Can you work these out from the model? Positions are in its coordinate system, mm. A direction names the side the tool comes from. Round coordinates to 2 decimals unless told otherwise and drop trailing zeros. Write each loop counter-clockwise with the first axis right and the second up, starting at its lowest first coordinate (ties: lowest second). Pieces come first, ordered by that corner, then holes. Notation, with made-up numbers: M 15.25,63.25 L 30.25,63.25 A16 cw 30.25,94.25 Z; hole C 84,31.25 d3. An arc over 180 degrees is marked long. Answer as a JSON object with one key per item and string values. Group by question number.
1) Please list where these lines run through material, in increasing order: L1, parallel to Z at x = -8, y = 4.3; L2, parallel to X at y = 3.25, z = -18.5. Write a range as [from, to].
2) If we mould it in two halves opening along X, with no side actions, what happens to faces 3 (the flat face through (-113.919, 3, 1)), 4 (the flat face through (108.839, 3, 1)), 5 (the flat face through (-9, 0, 79))? For each: +X half, -X half, draft (parallel to the pull), parting line (faces both ways), or undercut.
3) Suppose I cut it at B-B, the plane z = -10. Write out the boundary of the cut face in (x, y).
4) On a 3-axis mill with a long thin cutter (end or side, diameter ignored), from which of +Z, -Z, +X, -X, +Y, -Y can I reach the whole of each face in a straight line? I mean faces 1 (the flat face through (-9, 5.08, 79)), 2 (the cylindrical face through (-107.21, 2.58, 75.55)). Say none if no direction works.
5) Suppose I cut it at A-A, the plane x = 4. Write out the boundary of the cut face in (y, z), and give its area (3 significant figures).
6) Suppose I cut it at C-C, the plane y = 4.3. Write out the boundary of the cut face in (x, z), and give its area (3 significant figures).
from build123d import *

# Parameters (mm, degrees)
SKETCH1_W      = 227.838
SKETCH1_H      = 164.338
SKETCH1_W_2    = 217.678
SKETCH1_H_2    = 154.178
EXTRUDE1_DEPTH = 5.08
FILLET1_R      = 5.4102
FILLET2_R      = 10.4902


with BuildPart() as part:
    # Sketch1 → Extrude1 (new body)
    with BuildSketch(Plane(origin=(0, 0, 0), x_dir=(1, 0, 0), z_dir=(0, 1, 0))):
        Rectangle(SKETCH1_W, SKETCH1_H)
        Rectangle(SKETCH1_W_2, SKETCH1_H_2, mode=Mode.SUBTRACT)
    extrude(amount=EXTRUDE1_DEPTH)

    # Fillet1
    fillet1_edges = [part.edges().sort_by_distance(p)[0] for p in [
        (-108.839, 2.54, -77.089),
        (-108.839, 2.54, 77.089),
        (108.839, 2.54, 77.089),
        (108.839, 2.54, -77.089),
    ]]
    fillet(fillet1_edges, radius=FILLET1_R)

    # Fillet2
    fillet2_edges = [part.edges().sort_by_distance(p)[0] for p in [
        (-113.919, 2.54, -82.169),
        (113.919, 2.54, -82.169),
        (113.919, 2.54, 82.169),
        (-113.919, 2.54, 82.169),
    ]]
    fillet(fillet2_edges, radius=FILLET2_R)


solid = part.part
Results:
{
 "1": {"L1": "[-82.17, -77.09], [77.09, 82.17]", "L2": "[-113.92, -108.84], [108.84, 113.92]"},
 "2": {"face 3": "-X half", "face 4": "undercut", "face 5": "draft"},
 "3": {"outline": "M -113.92,0 L -108.84,0 L -108.84,5.08 L -113.92,5.08 Z; M 108.84,0 L 113.92,0 L 113.92,5.08 L 108.84,5.08 Z"},
 "4": {"face 1": "+Z, -Z, +X, -X, +Y", "face 2": "+Y, -Y"},
 "5": {"outline": "M 0,-82.17 L 5.08,-82.17 L 5.08,-77.09 L 0,-77.09 Z; M 0,77.09 L 5.08,77.09 L 5.08,82.17 L 0,82.17 Z", "area": "51.6 mm^2"},
 "6": {"outline": "M -113.92,-71.68 A10.49 ccw -103.43,-82.17 L 103.43,-82.17 A10.49 ccw 113.92,-71.68 L 113.92,71.68 A10.49 ccw 103.43,82.17 L -103.43,82.17 A10.49 ccw -113.92,71.68 Z; hole M -108.84,-71.68 A5.41 ccw -103.43,-77.09 L 103.43,-77.09 A5.41 ccw 108.84,-71.68 L 108.84,71.68 A5.41 ccw 103.43,77.09 L -103.43,77.09 A5.41 ccw -108.84,71.68 Z", "area": "3,810 mm^2"}
}
